Geometry check sheet. Reference: the model listing, model coordinates, mm. A direction names the side the tool comes from. Give positions to 0.01 mm unless a question says otherwise; leave off trailing zeros. Order: outer loops, then holes, each group sorted by start corner. A loop starts at its lowest first (then second) coordinate and runs counter-clockwise, first axis right, second up. Notation, with made-up numbers: (-7, -18.75) - (-1, -18.75) arc R19 ccw to (-1, 3.25) - close; hole circle Ø5 at (-19, 68). An arc over 180 degrees is marked (long way). Put each result on its own line as item: value. Start each with the question number.
```python
from build123d import *

# Parameters (mm, degrees)
SKETCH1_W           = 134.62
SKETCH1_H           = 134.62
BOSS_EXTRUDE1_DEPTH = 144.78
FILLET1_R           = 58.42
FILLET2_R           = 10.16
SKETCH2_R           = 55.88
BOSS_EXTRUDE2_DEPTH = 21.59
SHELL1_T            = -7.62


with BuildPart() as part:
    # Sketch1 → Boss-Extrude1 (new body)
    with BuildSketch(Plane(origin=(0, 0, 0), x_dir=(1, 0, 0), z_dir=(0, 1, 0))):
        Rectangle(SKETCH1_W, SKETCH1_H)
    extrude(amount=BOSS_EXTRUDE1_DEPTH)

    # Fillet1
    fillet1_edges = [part.edges().sort_by_distance(p)[0] for p in [
        (67.31, 72.39, 67.31),
        (-67.31, 72.39, 67.31),
        (-67.31, 72.39, -67.31),
        (67.31, 72.39, -67.31),
    ]]
    fillet(fillet1_edges, radius=FILLET1_R)

    # Fillet2
    fillet2_edges = [part.edges().sort_by_distance(p)[0] for p in [
        (67.31, 0, 0),
        (67.31, 144.78, 0),
        (0, 0, 67.31),
        (-67.31, 0, 0),
        (0, 0, -67.31),
        (-50.199178157, 0, -50.199178157),
        (50.199178157, 0, -50.199178157),
        (-50.199178157, 0, 50.199178157),
        (50.199178157, 0, 50.199178157),
        (0, 144.78, 67.31),
        (0, 144.78, -67.31),
        (-67.31, 144.78, 0),
        (-50.199178157, 144.78, -50.199178157),
        (50.199178157, 144.78, -50.199178157),
        (-50.199178157, 144.78, 50.199178157),
        (50.199178157, 144.78, 50.199178157),
    ]]
    fillet(fillet2_edges, radius=FILLET2_R)

    # Sketch2 → Boss-Extrude2 (add)
    with BuildSketch(Plane(origin=(0, 144.78, 0), x_dir=(1, 0, 0), z_dir=(0, 1, 0))):
        with Locations(Location((0, 0, 0), (0, 0, 270))):
            Circle(SKETCH2_R)
    extrude(amount=BOSS_EXTRUDE2_DEPTH)

    # Shell1
    shell1_openings = [part.faces().sort_by_distance(p)[0] for p in [
        (0, 166.37, 0),
    ]]
    offset(amount=SHELL1_T, openings=shell1_openings, kind=Kind.INTERSECTION)


solid = part.part
```
Item 1: Cross-section at A-A (y = 116). Enter the section's corners in (x, z).
Item 2: Thickness scan on line 1 along X through (y, z) = (147.5, 0); line 2 along X through (y, z) = (17, -5.5); line 3 along Y through (x, z) = (48.5, -21). Record the ranges inside material, lowest first.
Item 3: Set-up check for faces 1 (the face through (0.124, 141.883, 64.255)), 2 (the face through (-59.69, 72, 0)), 3 (the face through (14.5, 151.56, 46.03)): record each of +Z, -Z, +X, -X, +Y, -Y from which the full face is reachable in a straight line by a thin tool's end or side.
Item 4: Cross-section at C-C (z = 0). Enter the section's corners in (x, y).
Item 5: Cross-section at B-B (x = 0). Enter the section's corners in (y, z), and give its area (3 significant figures).
Item 6: Gauge pin test, flat ends, axial feed: pin 1 Ø10 at (x, y) = (-16, 58.5) entering from +Z; pin 2 Ø12 at (x, z) = (-30.5, -29) entering from +Y; pin 3 Ø2 at (y, z) = (70.5, 24) entering from +X. Record the tip position at first contact, or that the pin passes through.
Item 7: Release check for a two-part mould opening along Y. For faces 4 (the face through (55.4, 155.4, -7.3)), 5 (the face through (-47, 137.16, 12)), 6 (the face through (-55, 144.78, -13)) record: +Y half, -Y half, draft (parallel to the pull), parting line (faces both ways), or undercut.
Recorded:
1. outline: (-67.31, -8.89) arc R58.42 ccw to (-8.89, -67.31) - (8.89, -67.31) arc R58.42 ccw to (67.31, -8.89) - (67.31, 8.89) arc R58.42 ccw to (8.89, 67.31) - (-8.89, 67.31) arc R58.42 ccw to (-67.31, 8.89) - close; hole (-59.69, -8.89) arc R50.8 ccw to (-8.89, -59.69) - (8.89, -59.69) arc R50.8 ccw to (59.69, -8.89) - (59.69, 8.89) arc R50.8 ccw to (8.89, 59.69) - (-8.89, 59.69) arc R50.8 ccw to (-59.69, 8.89) - close
2. line 1: x = -55.88 to -48.26, 48.26 to 55.88
2. line 2: x = -67.31 to -59.69, 59.69 to 67.31
2. line 3: y = 0 to 7.62, 137.16 to 166.37
3. face 1: +Z, +X, -X, +Y
3. face 2: none
3. face 3: +Y
4. outline: (-67.31, 10.16) arc R10.16 ccw to (-57.15, 0) - (57.15, 0) arc R10.16 ccw to (67.31, 10.16) - (67.31, 134.62) arc R10.16 ccw to (57.15, 144.78) - (55.88, 144.78) - (55.88, 166.37) - (48.26, 166.37) - (48.26, 137.16) - (57.15, 137.16) arc R2.54 cw to (59.69, 134.62) - (59.69, 10.16) arc R2.54 cw to (57.15, 7.62) - (-57.15, 7.62) arc R2.54 cw to (-59.69, 10.16) - (-59.69, 134.62) arc R2.54 cw to (-57.15, 137.16) - (-48.26, 137.16) - (-48.26, 166.37) - (-55.88, 166.37) - (-55.88, 144.78) - (-57.15, 144.78) arc R10.16 ccw to (-67.31, 134.62) - close
5. outline: (0, -57.15) arc R10.16 ccw to (10.16, -67.31) - (134.62, -67.31) arc R10.16 ccw to (144.78, -57.15) - (144.78, -55.88) - (166.37, -55.88) - (166.37, -48.26) - (137.16, -48.26) - (137.16, -57.15) arc R2.54 cw to (134.62, -59.69) - (10.16, -59.69) arc R2.54 cw to (7.62, -57.15) - (7.62, 57.15) arc R2.54 cw to (10.16, 59.69) - (134.62, 59.69) arc R2.54 cw to (137.16, 57.15) - (137.16, 48.26) - (166.37, 48.26) - (166.37, 55.88) - (144.78, 55.88) - (144.78, 57.15) arc R10.16 ccw to (134.62, 67.31) - (10.16, 67.31) arc R10.16 ccw to (0, 57.15) - close
5. area: 3,540 mm^2
6. pin 1: stops at z = 67.27
6. pin 2: stops at y = 7.62
6. pin 3: stops at x = 65.58
7. face 4: draft
7. face 5: undercut
7. face 6: +Y half
